Check sheet for the drawn part. Datum: minimum x, y, z corner. Units: mm. A direction names the side the tool comes from. Coordinates: 2 decimals unless noted, no trailing zeros. Loops run counter-clockwise (first coordinate to the right, second up) from the corner with the lowest first, then second, coordinate; pieces in that order, holes last. Notation, with made-up numbers: M 50,70.25 L 71,70.25 A22 ccw 71,80.25 Z; hole C -15,48.25 d7. An arc over 180 degrees is marked long. Answer as CSV lines item,"result". Start each with the question number.
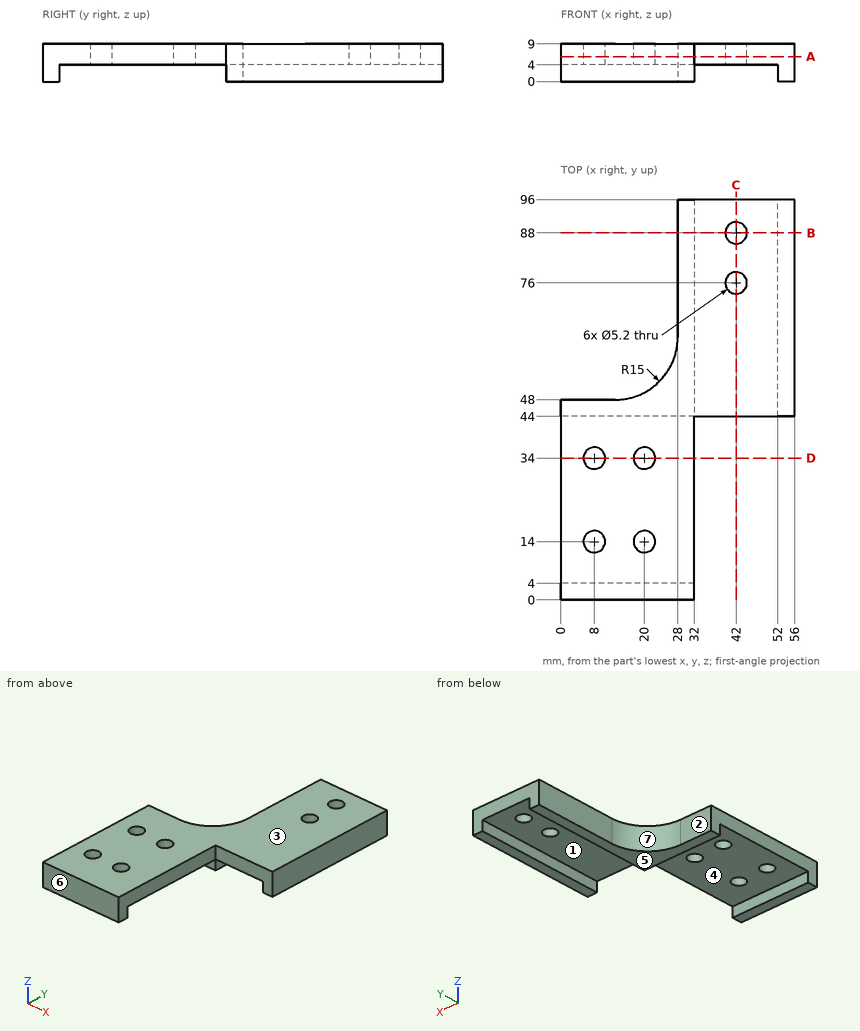
Item 1: Sectioned sample at B-B, the plane y = 88. Record the boundary of the cut face in (x, z), and give its area (3 significant figures).
Item 2: Go/stop test with flat-tipped pins: pin 1 (3 mm diameter, centred on x = 13, z = 2, fed in from +Y); pin 2 (6 mm diameter, centred on x = 42, y = 76, fed in from +Z); pin 3 (1 mm diameter, centred on x = 40.5, y = 56, fed in from -Z); pin 4 (2.5 mm diameter, centred on y = 78, z = 3.5, fed in from -X). Record where each tip stops, or that it passes through.
Item 3: Sectioned sample at A-A, the plane z = 6. Record the boundary of the cut face in (x, y), and give its area (3 significant figures).
Item 4: Sectioned sample at C-C, the plane x = 42. Record the boundary of the cut face in (y, z).
Item 5: Sectioned sample at D-D, the plane y = 34. Record the boundary of the cut face in (x, z).
Item 6: Material ranges on line 1 (Y direction, x = 42, z = 6.15); line 2 (X direction, y = 69, z = 3.25); line 3 (Y direction, x = 44, z = 8.5), recorded low to high. Write a range as from..to.
Item 7: Set-up check for the marked faces 1, 2 and 3: record each of +Z, -Z, +X, -X, +Y, -Y from which the full face is reachable in a straight line by a thin tool's end or side.
Item 8: Release check for a two-part mould opening along Y. For the marked faces 4, 5, 6 and 7 record: released by +Y, released by -Y, zero draft, split by the parting line, or undercut.
Reply:
1,outline,"M 28,0 L 32,0 L 32,4 L 39.4,4 L 39.4,9 L 28,9 Z; M 44.6,4 L 52,4 L 52,0 L 56,0 L 56,9 L 44.6,9 Z"
1,area,"146 mm²"
2,pin 1,"y = 48.08"
2,pin 2,"z = 9"
2,pin 3,"z = 4"
2,pin 4,"x = 28"
3,outline,"M 0,0 L 32,0 L 32,44 L 56,44 L 56,96 L 28,96 L 28,63 A15 cw 13,48 L 0,48 Z; hole C 8,14 d5.2; hole C 8,34 d5.2; hole C 20,14 d5.2; hole C 20,34 d5.2; hole C 42,76 d5.2; hole C 42,88 d5.2"
3,area,"2,900 mm²"
4,outline,"M 44,4 L 73.4,4 L 73.4,9 L 44,9 Z; M 78.6,4 L 85.4,4 L 85.4,9 L 78.6,9 Z; M 90.6,4 L 96,4 L 96,9 L 90.6,9 Z"
5,outline,"M 0,4 L 5.4,4 L 5.4,9 L 0,9 Z; M 10.6,4 L 17.4,4 L 17.4,9 L 10.6,9 Z; M 22.6,4 L 32,4 L 32,9 L 22.6,9 Z"
6,line 1,"44..73.4, 78.6..85.4, 90.6..96"
6,line 2,"28..32, 52..56"
6,line 3,"44..74.34, 77.66..86.34, 89.66..96"
7,face 1,"-Z, +Y, -Y"
7,face 2,"+Z, -Z, -X, +Y"
7,face 3,"+Z, +X, -X, +Y, -Y"
8,face 4,"undercut"
8,face 5,"zero draft"
8,face 6,"released by -Y"
8,face 7,"released by +Y"
